from build123d import *

# Parameters (mm, degrees)
SKETCH1_W                 = 20
SKETCH1_H                 = 30
BOSS_EXTRUDE1_DEPTH       = 183.3
SKETCH13_W                = 30
SKETCH13_H                = 57
BOSS_EXTRUDE2_DEPTH       = 11
SKETCH3_W                 = 20.6
SKETCH3_H                 = 41
CUT_EXTRUDE1_DEPTH        = 40
SKETCH11_R                = 10.5
CUT_EXTRUDE4_DEPTH        = 2.4
SKETCH12_R                = 4
CUT_EXTRUDE5_DEPTH        = 185.752943143
SKETCH14_W                = 31
SKETCH14_H                = 41
CUT_EXTRUDE6_DEPTH        = 25.3
F_2_CLEARANCE_HOLE2_D     = 2.4384
F_2_CLEARANCE_HOLE2_DEPTH = 6.35
F_2_CLEARANCE_HOLE2_TIP   = 0.732569267
CUT_EXTRUDE8_START        = -2
CUT_EXTRUDE8_DEPTH        = 1.6
F_2_CLEARANCE_HOLE3_D     = 2.4384
F_2_CLEARANCE_HOLE3_DEPTH = 6.35
F_2_CLEARANCE_HOLE3_TIP   = 0.732569267
FILLET3_R                 = 15
FILLET4_R                 = 5
FILLET5_R                 = 2
SKETCH21_W                = 6
SKETCH21_H                = 10
CUT_EXTRUDE9_DEPTH        = 8
FILLET6_R                 = 12
FILLET7_R                 = 6
CUT_EXTRUDE10_START       = -2
CUT_EXTRUDE10_DEPTH       = 1.9


# Some blends are built 0.0001 mm under size
with BuildPart() as part:
    # Sketch1 → Boss-Extrude1 (new body)
    with BuildSketch(Plane(origin=(0, 0, 0), x_dir=(1, 0, 0), z_dir=(0, 1, 0))):
        Rectangle(SKETCH1_W, SKETCH1_H)
    extrude(amount=BOSS_EXTRUDE1_DEPTH)

    # Sketch13 → Boss-Extrude2 (add)
    with BuildSketch(Plane.ZY.offset(-10)):
        with Locations((0, 28.5)):
            Rectangle(SKETCH13_W, SKETCH13_H)
    extrude(amount=-BOSS_EXTRUDE2_DEPTH)

    # Sketch3 → Cut-Extrude1 (cut)
    with BuildSketch(Plane(origin=(21, 0, 0), x_dir=(0, 0, -1), z_dir=(1, 0, 0))):
        with Locations((0, 28.5)):
            Rectangle(SKETCH3_W, SKETCH3_H)
    extrude(amount=-CUT_EXTRUDE1_DEPTH, mode=Mode.SUBTRACT)

    # Sketch11 → Cut-Extrude4 (cut)
    with BuildSketch(Plane.ZY.offset(-10)):
        with Locations((0, 168.3)):
            Circle(SKETCH11_R)
    extrude(amount=CUT_EXTRUDE4_DEPTH, mode=Mode.SUBTRACT)

    # Sketch12 → Cut-Extrude5 (cut, through all)
    with BuildSketch(Plane(origin=(7.6, 0, 0), x_dir=(0, 0, -1), z_dir=(1, 0, 0))):
        with Locations((0, 168.3)):
            Circle(SKETCH12_R)
    extrude(amount=-CUT_EXTRUDE5_DEPTH, mode=Mode.SUBTRACT)

    # Sketch14 → Cut-Extrude6 (cut)
    with BuildSketch(Plane(origin=(0, 0, -15), x_dir=(-1, 0, 0), z_dir=(0, 0, -1))):
        with Locations((-5.5, 28.5)):
            Rectangle(SKETCH14_W, SKETCH14_H)
    extrude(amount=-CUT_EXTRUDE6_DEPTH, mode=Mode.SUBTRACT)

    # #2 Clearance Hole2
    with Locations(Plane(origin=(21, 0, 0), x_dir=(0, 0, -1), z_dir=(1, 0, 0))):
        with Locations((-7.5, 5), (9.5, 5), (-7.5, 52), (9.5, 52)):
            Hole(F_2_CLEARANCE_HOLE2_D / 2, depth=F_2_CLEARANCE_HOLE2_DEPTH)
            with Locations((0, 0, -(F_2_CLEARANCE_HOLE2_DEPTH + F_2_CLEARANCE_HOLE2_TIP / 2))):  # 118° drill point
                Cone(0, F_2_CLEARANCE_HOLE2_D / 2, F_2_CLEARANCE_HOLE2_TIP, mode=Mode.SUBTRACT)

    # Sketch18 → Cut-Extrude8 (cut)
    with BuildSketch(Plane(origin=(21, 0, 0), x_dir=(0, 0, -1), z_dir=(1, 0, 0)).offset(CUT_EXTRUDE8_START)):
        Polygon((-10.329016319, 5), (-8.91450816, 2.55), (-6.08549184, 2.55), (-4.670983681, 5), (-6.08549184, 7.45), (-8.91450816, 7.45), align=None)
        Polygon((12.329016319, 5), (10.91450816, 7.45), (8.08549184, 7.45), (6.670983681, 5), (8.08549184, 2.55), (10.91450816, 2.55), align=None)
        Polygon((6.670983681, 52), (8.08549184, 49.55), (10.91450816, 49.55), (12.329016319, 52), (10.91450816, 54.45), (8.08549184, 54.45), align=None)
        Polygon((-4.670983681, 52), (-6.08549184, 54.45), (-8.91450816, 54.45), (-10.329016319, 52), (-8.91450816, 49.55), (-6.08549184, 49.55), align=None)
    extrude(amount=-CUT_EXTRUDE8_DEPTH, mode=Mode.SUBTRACT)

    # #2 Clearance Hole3
    with Locations(Plane(origin=(-10, 0, 0), x_dir=(0, 0, -1), z_dir=(-1, 0, 0))):
        with Locations((8.22, -4.1), (-3.52, -4.1), (-3.52, -52.9), (8.22, -52.9)):
            Hole(F_2_CLEARANCE_HOLE3_D / 2, depth=F_2_CLEARANCE_HOLE3_DEPTH)
            with Locations((0, 0, -(F_2_CLEARANCE_HOLE3_DEPTH + F_2_CLEARANCE_HOLE3_TIP / 2))):  # 118° drill point
                Cone(0, F_2_CLEARANCE_HOLE3_D / 2, F_2_CLEARANCE_HOLE3_TIP, mode=Mode.SUBTRACT)

    # Fillet3
    fillet3_edges = [part.edges().sort_by_distance(p)[0] for p in [
        (0, 183.3, 15),
        (0, 183.3, -15),
    ]]
    fillet(fillet3_edges, radius=FILLET3_R - 0.0001)  # a hair under: the kernel refuses the full size

    # Fillet4
    fillet4_edges = [part.edges().sort_by_distance(p)[0] for p in [
        (15.5, 57, -15),
        (15.5, 57, 15),
        (5.5, 0, -15),
        (5.5, 0, 15),
    ]]
    fillet(fillet4_edges, radius=FILLET4_R)

    # Fillet5
    fillet5_edges = [part.edges().sort_by_distance(p)[0] for p in [
        (10, 110.15005, 15),
        (10, 110.15005, -15),
        (10, 178.906631007, -10.606631007),
        (10, 178.906631007, 10.606631007),
        (-10, 86.65005, 15),
        (-10, 108.65005, -15),
        (-10, 178.906631007, -10.606631007),
        (-10, 178.906631007, 10.606631007),
        (-10, 0, 0),
        (-10, 1.464466094, -13.535533906),
        (-10, 1.464466094, 13.535533906),
        (-10, 6.5, -15),
    ]]
    fillet(fillet5_edges, radius=FILLET5_R)

    # Sketch21 → Cut-Extrude9 (cut)
    with BuildSketch(Plane.XZ):
        with Locations((13.5, 0)):
            Rectangle(SKETCH21_W, SKETCH21_H)
    extrude(amount=-CUT_EXTRUDE9_DEPTH, mode=Mode.SUBTRACT)

    # Fillet6
    # the kernel refuses this fillet: 12 mm, written as the material it takes off along each edge
    with BuildSketch(Plane(origin=(10.5, 8, 5), x_dir=(-1, 0, 0), z_dir=(0, 0, -1))) as fillet6_piece_1:
        with BuildLine():
            CenterArc((11.313708499, -12), FILLET6_R, 90, 70.528779366)
            Line((0, -8), (0, 0))
            Line((0, 0), (11.313708499, 0))
        make_face()
    extrude(amount=10, mode=Mode.SUBTRACT)

    # Fillet7
    # the kernel refuses this fillet: 6 mm, written as the material it takes off along each edge
    with BuildSketch(Plane(origin=(16.5, 0, 5), x_dir=(0, 1, 0), z_dir=(-1, 0, 0))) as fillet7_piece_1_section:
        with BuildLine():
            CenterArc((FILLET7_R, -FILLET7_R), FILLET7_R, 90, 90)
            Line((0, -FILLET7_R), (0, 0))
            Line((0, 0), (FILLET7_R, 0))
        make_face()
    fillet7_piece_1 = extrude(amount=21, mode=Mode.PRIVATE)
    fillet7_piece_1 = fillet7_piece_1 - Plane(origin=(-0.813708499, -4, 5.004149899), x_dir=(-1, 0, 0), z_dir=(0, 0, 1)) * Cylinder(12, 66, mode=Mode.PRIVATE)
    add(fillet7_piece_1, mode=Mode.SUBTRACT)

    # Sketch22 → Cut-Extrude10 (cut)
    with BuildSketch(Plane.ZY.offset(10).offset(CUT_EXTRUDE10_START)):
        Polygon((0.690983681, 52.9), (2.10549184, 50.45), (4.93450816, 50.45), (6.349016319, 52.9), (4.93450816, 55.35), (2.10549184, 55.35), align=None)
        Polygon((-11.049016319, 52.9), (-9.63450816, 50.45), (-6.80549184, 50.45), (-5.390983681, 52.9), (-6.80549184, 55.35), (-9.63450816, 55.35), align=None)
        Polygon((-5.390983681, 4.1), (-6.80549184, 6.55), (-9.63450816, 6.55), (-11.049016319, 4.1), (-9.63450816, 1.65), (-6.80549184, 1.65), align=None)
        Polygon((6.349016319, 4.1), (4.93450816, 6.55), (2.10549184, 6.55), (0.690983681, 4.1), (2.10549184, 1.65), (4.93450816, 1.65), align=None)
    extrude(amount=-CUT_EXTRUDE10_DEPTH, mode=Mode.SUBTRACT)


solid = part.part
Geometry check sheet. Reference: the model listing, model coordinates, mm. A direction names the side the tool comes from. Round coordinates to 2 decimals unless told otherwise and drop trailing zeros. Write each loop counter-clockwise with the first axis right and the second up, starting at its lowest first coordinate (ties: lowest second). Pieces come first, ordered by that corner, then holes. Notation, with made-up numbers: (-4, 62.5) -> (22, 62.5) arc R33 ccw to (22, 92.5) -> close; hole circle Ø2 at (60, 77). An arc over 180 degrees is marked (long way). One line per item, written item: value. Start each with the question number.
(1) Draft check along X on faces 5 (the cylindrical face through (15, 55, -14)), 6 (the flat face through (19, 6, 6)), 7 (the flat face through (21, 29, 11)). Enter one of: +X half, -X half, draft (parallel to the pull), parting line (faces both ways), or undercut.
(2) Go/stop test with flat-tipped pins: pin 1 Ø0.5 at (x, z) = (18, 8) entering from +Y; pin 2 Ø6 at (y, z) = (65, -9) entering from +X; pin 3 Ø5.5 at (y, z) = (53, 3.5) entering from -X; pin 4 Ø1 at (x, z) = (-6.5, 4) entering from +Y. Record where each tip stops, or that it passes through.
(3) Cross-section at B-B, the plane y = 12. Record the cut outline in (x, z), and give its area (3 significant figures).
(4) Access from +Z, -Z, +X, -X, +Y, -Y to the whole of each face (thin tool, end or side, straight path). Record for faces 1 (the flat face through (6, 28, 10.3)), 2 (the cylindrical face through (8.82, 158.05, -2.28)), 3 (the flat face through (12, 5, -5)), 4 (the cylindrical face through (15, 55, 14)).
(5) Cross-section at A-A, the plane y = 74. Record the cut outline in (x, z), and give its area (3 significant figures).
(6) Scan lines: line 1 (Z direction, x = -5.2, y = 4.1); line 2 (Y direction, x = 6.5, z = 1.5); line 3 (Z direction, x = 8, y = 168). Record each from-to range of solid material in increasing order. Write a range as [from, to].
Answer:
1. face 5: draft
1. face 6: undercut
1. face 7: +X half
2. pin 1: y = 57
2. pin 2: x = 10
2. pin 3: x = -10
2. pin 4: y = 182.89
3. outline: (-10, 10.3) -> (21, 10.3) -> (21, 15) -> (-8, 15) arc R2 ccw to (-10, 13) -> close
3. area: 145 mm²
4. face 1: -Z, +X, -X
4. face 2: +X
4. face 3: none
4. face 4: +Z, +X, +Y
5. outline: (-10, -13) arc R2 ccw to (-8, -15) -> (8, -15) arc R2 ccw to (10, -13) -> (10, 13) arc R2 ccw to (8, 15) -> (-8, 15) arc R2 ccw to (-10, 13) -> close
5. area: 597 mm²
6. line 1: [-14.92, -9.44], [-7, 2.3], [4.74, 14.92]
6. line 2: [0, 5.51], [49, 164.59], [172.01, 183.22]
6. line 3: [-15, -10.5], [10.5, 15]
